Input: part model. Units: mm. Frame: model coordinates. Face numbers are marked on the shaded views. A direction names the side the tool comes from. Coordinates: 2 decimals unless noted, no trailing zeros. Order: outer loops, then holes, each group sorted by start corner. A loop starts at its lowest first (then second) coordinate and runs counter-clockwise, first axis right, second up. Notation, with made-up numbers: M 4,44.25 L 21,44.25 A22 cw 21,61.25 Z; hole C -30,-29 d11. An arc over 180 degrees is marked long. One line per item, written item: value.
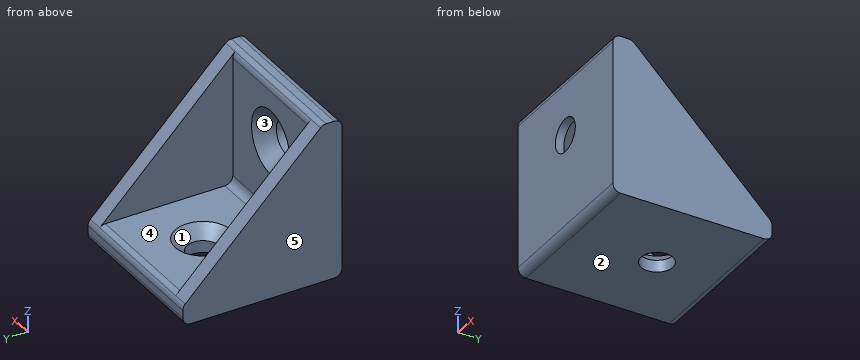
```python
from build123d import *

# Parameters (mm, degrees)
PAD_DEPTH            = 20
POCKET_DEPTH         = 16
HOLE_D               = 4
HOLE_CSINK_D         = 7
HOLE_CSINK_ANGLE     = 90
HOLE001_D            = 4.2
HOLE001_DEPTH        = 25
HOLE001_CSINK_D      = 8.1
HOLE001_CSINK_ANGLE  = 90
BODY_PLACEMENT_ANGLE = 90


with BuildPart() as part:
    # Sketch → Pad (new body)
    with BuildSketch(Plane.XZ):
        with BuildLine():
            Line((0, 19), (0, 1))
            ThreePointArc((0, 1), (0.292893, 0.292893), (1, 0))
            Line((1, 0), (19, 0))
            ThreePointArc((19, 0), (19.707107, 0.292893), (20, 1))
            Line((20, 1), (20, 2))
            ThreePointArc((20, 2), (19.92388, 2.382683), (19.707107, 2.707107))
            Line((19.707107, 2.707107), (2.707107, 19.707107))
            ThreePointArc((2.707107, 19.707107), (2.382683, 19.92388), (2, 20))
            Line((2, 20), (1, 20))
            ThreePointArc((1, 20), (0.292893, 19.707107), (0, 19))
        make_face()
    extrude(amount=PAD_DEPTH)

    # Sketch001 (on Face12 of Pad) → Pocket (cut)
    with BuildSketch(Plane.XZ.offset(18)):
        with BuildLine():
            Line((3, 19), (3, 4))
            ThreePointArc((3, 4), (3.292893, 3.292893), (4, 3))
            Line((4, 3), (19, 3))
            ThreePointArc((20, 2), (19.707107, 2.707107), (19, 3))
            Line((20, 20), (20, 2))
            Line((2, 20), (20, 20))
            ThreePointArc((3, 19), (2.707107, 19.707107), (2, 20))
        make_face()
    extrude(amount=-POCKET_DEPTH, mode=Mode.SUBTRACT)

    # Hole (through all)
    with Locations(Plane(origin=(0, 0, 3), x_dir=(-1, 0, 0), z_dir=(0, 0, 1))):
        with Locations((-11.5, 10)):
            CounterSinkHole(HOLE_D / 2, HOLE_CSINK_D / 2, counter_sink_angle=HOLE_CSINK_ANGLE)

    # Hole001
    with Locations(Plane(origin=(3, 0, 0), x_dir=(0, 0, 1), z_dir=(1, 0, 0))):
        with Locations((12.5, 10)):
            CounterSinkHole(HOLE001_D / 2, HOLE001_CSINK_D / 2, depth=HOLE001_DEPTH, counter_sink_angle=HOLE001_CSINK_ANGLE)


with BuildPart() as part_1:
    # Body placement: moved
    add(part.part.moved(Location((60, 13.9, 0))).rotate(Axis((60, 13.9, 0), (0, 0, 1)), BODY_PLACEMENT_ANGLE))


solid = part_1.part
```
(1) Cut plane D-D on x = 61.5. Output: boundary loops of the cut face in (y, z), plus the area to 3 significant figures.
Data:
outline: M 13.9,1 A1 ccw 14.9,0 L 32.9,0 A1 ccw 33.9,1 L 33.9,2 A1 ccw 33.61,2.71 L 16.61,19.71 A1 ccw 15.9,20 L 14.9,20 A1 ccw 13.9,19 Z
area: 245 mm2
(2) Cut plane A-A on x = 70. Output: boundary loops of the cut face in (y, z), plus the area to 3 significant figures.
Data:
outline: M 13.9,1 A1 ccw 14.9,0 L 23.4,0 L 23.4,1.5 L 21.9,3 L 17.9,3 A1 cw 16.9,4 L 16.9,8.45 L 14.95,10.4 L 13.9,10.4 Z; M 13.9,14.6 L 14.95,14.6 L 16.9,16.55 L 16.9,19 A1 ccw 15.9,20 L 14.9,20 A1 ccw 13.9,19 Z; M 27.4,0 L 32.9,0 A1 ccw 33.9,1 L 33.9,2 A1 ccw 32.9,3 L 28.9,3 L 27.4,1.5 Z
area: 79.5 mm2
(3) Draft query along Y for the marked faces 1, 2 and 3. Return one class per face: released by +Y, released by -Y, zero draft, split by the parting line, or undercut.
Data:
face 1: undercut
face 2: zero draft
face 3: released by +Y
(4) Ray query, line 1 (X direction, y = 14.75, z = 12.5); line 2 (X direction, y = 25.4, z = 1.1); line 3 (Y direction, x = 70, z = 1.05). Return the intervals inside material, ascending. Write a range as from..to.
Data:
line 1: x = 60..67.9, 72.1..80
line 2: x = 60..68, 72..80
line 3: y = 13.9..23.4, 27.4..33.9
(5) First-contact query: pin 1 (2 mm diameter, centred on x = 72, y = 27, fed in from +Z); pin 2 (5 mm diameter, centred on x = 70, z = 12.5, fed in from +Y); pin 3 (7.5 mm diameter, centred on x = 73, z = 12, fed in from +Y); pin 4 (2.5 mm diameter, centred on x = 70, y = 25.4, fed in from -Z). Flat tips, straight axial feed; report the tip coordinate or a pass-through.
Data:
pin 1: stops at z = 3
pin 2: stops at y = 15.35
pin 3: stops at y = 16.9
pin 4: passes through
(6) Access query for the marked faces 4 and 5. Directions: +Z, -Z, +X, -X, +Y, -Y. A direction counts if a zero-diameter tool reaches every point of the face in a straight line with its end or side. Return the directions, or none.
Data:
face 4: +Z, +Y
face 5: +Z, -Z, -X, +Y, -Y
(7) Cut plane C-C on z = 12.5. Output: boundary loops of the cut face in (x, y), plus the area to 3 significant figures.
Data:
outline: M 60,13.9 L 67.9,13.9 L 67.9,14.95 L 65.95,16.9 L 62,16.9 L 62,23.81 L 60,23.81 Z; M 72.1,13.9 L 80,13.9 L 80,23.81 L 78,23.81 L 78,16.9 L 74.05,16.9 L 72.1,14.95 Z
area: 71.3 mm2
(8) Cut plane B-B on y = 25.4. Output: boundary loops of the cut face in (x, z), plus the area to 3 significant figures.
Data:
outline: M 60,0 L 68,0 L 68,1.5 L 66.5,3 L 62,3 L 62,10.91 L 60,10.91 Z; M 72,0 L 80,0 L 80,10.91 L 78,10.91 L 78,3 L 73.5,3 L 72,1.5 Z
area: 77.4 mm2
